Can you work these out from the model? Positions are in its coordinate system, mm. Give positions to 0.01 mm unless a question says otherwise; leave off trailing zeros. Loops run counter-clockwise (first coordinate to the right, second up) from the corner with the lowest first, then second, coordinate; pieces in that order, holes last. Notation, with made-up numbers: (52, 6) -> (108, 6) arc R29 ccw to (108, 45) -> close; hole circle Ø4 at (37.5, 43). An arc over 180 degrees is marked (long way). One line per question, with ' | ' between items.
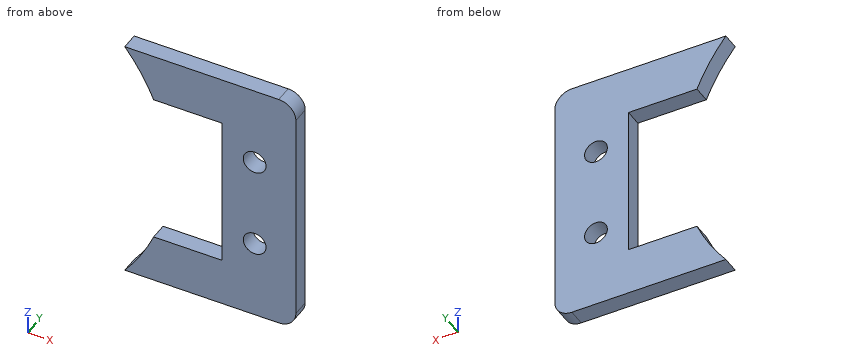
from build123d import *

# Parameters (mm, degrees)
SKETCH_1_R      = 2
EXTRUDE_1_DEPTH = 3
FILLET_1_R      = 3


with BuildPart() as part:
    # 草图1 → 凸台-拉伸1 (new body)
    with BuildSketch(Plane(origin=(0, 0, 0), x_dir=(1, 0, 0), z_dir=(0, 1, 0))):
        with BuildLine():
            Line((57.221315178, 22), (27.221315178, 22))
            ThreePointArc((27.221315178, 22), (30.058450594, 17.930129612), (32.291639785, 13.5))
            Line((32.291639785, 13.5), (44.291639785, 13.5))
            Line((44.291639785, 13.5), (44.291639785, -13.5))
            Line((44.291639785, -13.5), (32.291639785, -13.5))
            ThreePointArc((32.291639785, -13.5), (30.058450594, -17.930129612), (27.221315178, -22))
            Line((27.221315178, -22), (57.221315178, -22))
            Line((57.221315178, -22), (57.221315178, 22))
        make_face()
        with Locations(Location((50, -8, 0), (0, 0, 270))):
            Circle(SKETCH_1_R, mode=Mode.SUBTRACT)
        with Locations(Location((50, 8, 0), (0, 0, 270))):
            Circle(SKETCH_1_R, mode=Mode.SUBTRACT)
    extrude(amount=EXTRUDE_1_DEPTH)

    # 圆角1
    fillet_1_edges = [part.edges().sort_by_distance(p)[0] for p in [
        (57.221315178, 1.5, -22),
        (57.221315178, 1.5, 22),
    ]]
    fillet(fillet_1_edges, radius=FILLET_1_R)


solid = part.part
Q1. If we section it at B-B (z = 8): Write out the boundary of the cut face in (x, y).
Entries:
outline: (44.29, 0) -> (48, 0) -> (48, 3) -> (44.29, 3) -> close; (52, 0) -> (57.22, 0) -> (57.22, 3) -> (52, 3) -> close
Q2. If I drill on probe 1 along Z at (x, y) = (44.25, 1.35); probe 2 along X at (y, z) = (1.65, 8); probe 3 along X at (y, z) = (2.45, -3.5), over which ranges is the centre line in solid material (lowest first)? Write a range as from..to.
Entries:
probe 1: -22..-13.5, 13.5..22 | probe 2: 44.29..48, 52..57.22 | probe 3: 44.29..57.22
Q3. If we section it at A-A (x = 50): Write out the boundary of the cut face in (y, z), plus the area to 3 significant figures.
Entries:
outline: (0, -22) -> (3, -22) -> (3, -10) -> (0, -10) -> close; (0, -6) -> (3, -6) -> (3, 6) -> (0, 6) -> close; (0, 10) -> (3, 10) -> (3, 22) -> (0, 22) -> close | area: 108 mm²
Q4. For pin 1 Ø3 at (x, z) = (44, -5.5) entering from +Y; pin 2 Ø1.5 at (y, z) = (1, 12.5) entering from -X, each with a flat end and sliding along its axis, tell me the tip position at first contact or that it passes through.
Entries:
pin 1: y = 3 | pin 2: x = 44.29
Q5. If we section it at D-D (z = -7.5): Write out the boundary of the cut face in (x, y).
Entries:
outline: (44.29, 0) -> (48.06, 0) -> (48.06, 3) -> (44.29, 3) -> close; (51.94, 0) -> (57.22, 0) -> (57.22, 3) -> (51.94, 3) -> close
Q6. If we section it at C-C (y = 0.65): Write out the boundary of the cut face in (x, z), plus the area to 3 significant figures.
Entries:
outline: (27.22, -22) -> (54.22, -22) arc R3 ccw to (57.22, -19) -> (57.22, 19) arc R3 ccw to (54.22, 22) -> (27.22, 22) arc R35 cw to (32.29, 13.5) -> (44.29, 13.5) -> (44.29, -13.5) -> (32.29, -13.5) arc R35 cw to start; hole circle Ø4 at (50, -8); hole circle Ø4 at (50, 8) | area: 782 mm²
